Build history of the part. All positions in model axes, mm. Round coordinates to 2 decimals unless told otherwise and drop trailing zeros. Write each loop counter-clockwise with the first axis right and the second up, starting at its lowest first coordinate (ties: lowest second). Pieces come first, ordered by that corner, then holes. Notation, with made-up numbers: (52.25, 3.5) - (64.25, 3.5) arc R13 cw to (64.25, 28.5) - close; hole circle Ø7 at (81, -13.75). An arc over 180 degrees is marked (long way). Answer as a JSON object with one key per item and string values. Group by question number.
Item 1: Slice it at B-B, the plane z = 0. List the corners of the cut face in (x, y) (3 decimals), then the cut area to 3 significant figures.
Item 2: Probe line 1 (X direction, y = 1.8, z = 1); line 2 (Z direction, x = 33, y = 0.35); line 3 (Z direction, x = 10, y = 1.8). List the from-to ranges inside material, lowest first. Write a range as from..to.
Item 3: Slice it at C-C, the plane y = 0.6. Give the number of separate pieces and of enclosed holes in the cut face, then the cut area to 3 significant figures.
Item 4: Slice it at D-D, the plane z = -33. List the corners of the cut face in (x, y) (3 decimals).
Item 5: Slice it at A-A, the plane x = -10. List the corners of the cut face in (y, z) (3 decimals), then the cut area to 3 significant figures.
Item 6: Flat gauge pin, fed straight in: pin 1 (23 mm diameter, centred on x = 0, z = 0, fed in from +Y). Where does the tip first touch, or does it go through?
from build123d import *

# Parameters (mm, degrees)
SKETCH1_R               = 14.2875
SKETCH1_R_2             = 14.28115
BOSS_EXTRUDE1_DEPTH     = 3.175
F_10_CLEARANCE_HOLE1_D  = 5.1054
F_1_4_CLEARANCE_HOLE1_D = 6.7564
CUT_EXTRUDE2_DEPTH      = 4.175
FILLET2_R               = 9.525


with BuildPart() as part:
    # Sketch1 → Boss-Extrude1 (new body)
    with BuildSketch(Plane(origin=(0, 0, 0), x_dir=(1, 0, 0), z_dir=(0, 1, 0))):
        with BuildLine():
            Line((85.884602434, 50.671947857), (-3.15409287, 44.337954375))
            ThreePointArc((-3.15409287, 44.337954375), (-44.45, 0), (-3.15409287, -44.337954375))
            Line((-3.15409287, -44.337954375), (85.884602434, -50.671947857))
            ThreePointArc((85.884602434, -50.671947857), (140.28928, 0), (85.884602434, 50.671947857))
        make_face()
        with Locations((89.48928, 0)):
            Circle(SKETCH1_R, mode=Mode.SUBTRACT)
        Circle(SKETCH1_R_2, mode=Mode.SUBTRACT)
    extrude(amount=BOSS_EXTRUDE1_DEPTH)

    # #10 Clearance Hole1 (through all)
    with Locations(Plane(origin=(0, 3.175, 0), x_dir=(1, 0, 0), z_dir=(0, 1, 0))):
        with Locations((0, 25.4), (25.4, 0), (0, -25.4), (-25.4, 0)):
            Hole(F_10_CLEARANCE_HOLE1_D / 2)

    # 1/4 Clearance Hole1 (through all)
    with Locations(Plane(origin=(0, 3.175, 0), x_dir=(1, 0, 0), z_dir=(0, 1, 0))):
        with Locations((54.56428, 34.925), (54.56428, -34.925), (114.88928, 25.4), (114.88928, -25.4), (-38.1, 0), (34.925, 34.314713318), (34.925, -34.314713318)):
            Hole(F_1_4_CLEARANCE_HOLE1_D / 2)

    # Sketch7 → Cut-Extrude2 (cut, through all)
    with BuildSketch(Plane(origin=(0, 3.175, 0), x_dir=(1, 0, 0), z_dir=(0, 1, 0))):
        Polygon((44.323, 47.715357826), (140.28928, 54.542162621), (140.28928, -54.542162621), (44.323, -47.715357826), align=None)
    extrude(amount=-CUT_EXTRUDE2_DEPTH, mode=Mode.SUBTRACT)

    # Fillet2
    fillet2_edges = [part.edges().sort_by_distance(p)[0] for p in [
        (44.323, 1.5875, -47.715357826),
        (44.323, 1.5875, 47.715357826),
    ]]
    fillet(fillet2_edges, radius=FILLET2_R)


solid = part.part
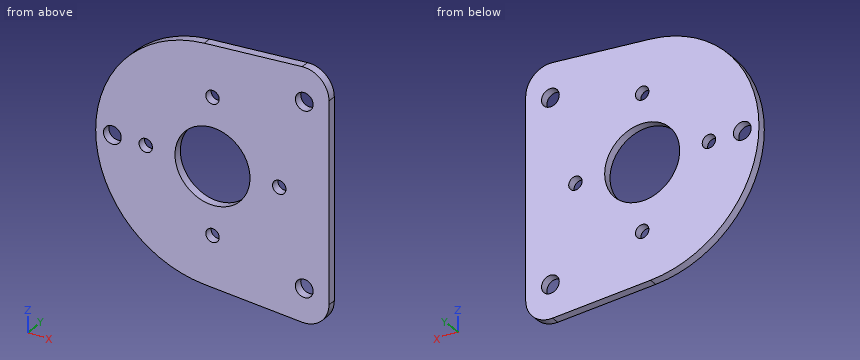
Geometry says:
{
 "1": {"outline": "(-44.45, 0) - (-41.478, 0) - (-41.478, 3.175) - (-44.45, 3.175) - close; (-34.722, 0) - (-27.953, 0) - (-27.953, 3.175) - (-34.722, 3.175) - close; (-22.847, 0) - (-14.281, 0) - (-14.281, 3.175) - (-22.847, 3.175) - close; (14.281, 0) - (22.847, 0) - (22.847, 3.175) - (14.281, 3.175) - close; (27.953, 0) - (44.323, 0) - (44.323, 3.175) - (27.953, 3.175) - close", "area": "137 mm^2"},
 "2": {"line 1": "x = -44.44..-41.33, -34.87..-27.75, -23.05..-14.25, 14.25..23.05, 27.75..44.32", "line 2": "z = -46.91..-37.09, -31.54..31.54, 37.09..46.91", "line 3": "z = -45.27..-10.2, 10.2..45.27"},
 "3": {"separate pieces": "1", "enclosed holes": "8", "area": "6,320 mm^2"},
 "4": {"outline": "(-29.779, 0) - (31.813, 0) - (31.813, 3.175) - (-29.779, 3.175) - close; (38.037, 0) - (44.323, 0) - (44.323, 3.175) - (38.037, 3.175) - close"},
 "5": {"outline": "(0, -43.311) - (3.175, -43.311) - (3.175, -10.196) - (0, -10.196) - close; (0, 10.196) - (3.175, 10.196) - (3.175, 43.311) - (0, 43.311) - close", "area": "210 mm^2"},
 "6": {"pin 1": "passes through"}
}
